```python
from build123d import *

# Parameters (mm, degrees)
SKETCH_1_W          = 24
SKETCH_1_H          = 27
EXTRUDE_1_DEPTH     = 33
SKETCH_3_W          = 24
SKETCH_3_H          = 25
CUT_EXTRUDE_1_DEPTH = 23


with BuildPart() as part:
    # 草图1 → 凸台-拉伸1 (new body)
    with BuildSketch(Plane(origin=(0, 0, 0), x_dir=(1, 0, 0), z_dir=(0, 1, 0))):
        Rectangle(SKETCH_1_W, SKETCH_1_H)
    extrude(amount=EXTRUDE_1_DEPTH)

    # 草图3 → 切除-拉伸1 (cut)
    with BuildSketch(Plane.XY.offset(13.5)):
        with Locations((0, 16.5)):
            Rectangle(SKETCH_3_W, SKETCH_3_H)
    extrude(amount=-CUT_EXTRUDE_1_DEPTH, mode=Mode.SUBTRACT)

    # 草图5 → M8 螺纹孔1 (revolve, cut)
    with BuildSketch(Plane(origin=(0, 16.5, -13.5), x_dir=(0, 1, 0), z_dir=(1, 0, 0))):
        Polygon((0, 0), (0, 4), (3.4, 4), (3.4, 0.625), (4.025, 0), align=None)
    revolve(axis=Axis((0, 16.5, -19.85), (0, 0, 1)), mode=Mode.SUBTRACT)


solid = part.part
```
The model under review builds one solid part; all positions refer to its coordinate system, in mm. A direction names the side the tool comes from. Round coordinates to 2 decimals unless told otherwise and drop trailing zeros. Loops run counter-clockwise (first coordinate to the right, second up) from the corner with the lowest first, then second, coordinate; pieces in that order, holes last. Notation, with made-up numbers: M -36.75,46 L 13.25,46 A11 cw 13.25,60 Z; hole C 63,7 d1. An arc over 180 degrees is marked long. Answer as a JSON object with one key per item and string values.
(1) Take a section at B-B on y = 16.5. Give the boundary of the cut face in (x, z) (3 decimals).
Resolved:
{"outline": "M -12,-13.5 L -4.025,-13.5 L -3.4,-12.875 L -3.4,-9.5 L -12,-9.5 Z; M 3.4,-12.875 L 4.025,-13.5 L 12,-13.5 L 12,-9.5 L 3.4,-9.5 Z"}
(2) Take a section at A-A on x = 0. Give the boundary of the cut face in (y, z) (3 decimals).
Resolved:
{"outline": "M 0,-13.5 L 12.475,-13.5 L 13.1,-12.875 L 13.1,-9.5 L 4,-9.5 L 4,13.5 L 0,13.5 Z; M 19.9,-12.875 L 20.525,-13.5 L 33,-13.5 L 33,13.5 L 29,13.5 L 29,-9.5 L 19.9,-9.5 Z"}
(3) To check wall thickness, follow line 1 along X through (y, z) = (16.5, -12.05); line 2 along Y through (x, z) = (5.25, 7); line 3 along Y through (x, z) = (0, -11.3). State the ranges of each line that lie inside material, in increasing order.
Resolved:
{"line 1": "-12 to -3.4, 3.4 to 12", "line 2": "0 to 4, 29 to 33", "line 3": "0 to 13.1, 19.9 to 33"}
(4) Draft analysis for pull direction X (two halves, no side actions). For faces 3 (the cylindrical face through (2.069, 13.802, -11.211)), 4 (the flat face through (-12, 16, -10)), 5 (the flat face through (0, 4, 2)), state which applies: released by +X, released by -X, zero draft, split by the parting line, or undercut.
Resolved:
{"face 3": "undercut", "face 4": "released by -X", "face 5": "zero draft"}
(5) Take a section at D-D on x = 5.5. Give the boundary of the cut face in (y, z).
Resolved:
{"outline": "M 0,-13.5 L 33,-13.5 L 33,13.5 L 29,13.5 L 29,-9.5 L 4,-9.5 L 4,13.5 L 0,13.5 Z"}
(6) Take a section at C-C on z = 3.25. Give the boundary of the cut face in (x, y), and give its area (3 significant figures).
Resolved:
{"outline": "M -12,0 L 12,0 L 12,4 L -12,4 Z; M -12,29 L 12,29 L 12,33 L -12,33 Z", "area": "192 mm²"}
(7) Clearance check with a flat-ended pin moving along its axis: P1, Ø12, axis at x = -2.5, z = -3, coming from the -Y side. State where the tip first meets the part, or that it passes through.
Resolved:
{"P1": "y = 0"}
(8) Tool access review of faces 1 (the flat face through (12, 16, -10)), 2 (the flat face through (2.5, 19.5, -9.5)): name each direction out of +Z, -Z, +X, -X, +Y, -Y from which nothing blocks a thin tool from reaching the whole face with its end or side.
Resolved:
{"face 1": "+Z, -Z, +X, +Y, -Y", "face 2": "+Z, +X, -X"}
